The listing builds one solid part. Answer for the finished solid, in the listing's coordinates (mm). A direction names the side the tool comes from. Round coordinates to 2 decimals unless told otherwise and drop trailing zeros. Loops run counter-clockwise (first coordinate to the right, second up) from the corner with the lowest first, then second, coordinate; pieces in that order, holes last. Notation, with made-up numbers: (31, 52) -> (78, 52) arc R10 ccw to (78, 57) -> close; hole circle Ø7 at (-6, 67.5). An arc over 180 degrees is marked (long way). One line per question, with ' | ' between items.
from build123d import *

# Parameters (mm, degrees)
SKETCH_1_W          = 23
SKETCH_1_H          = 12
EXTRUDE_1_DEPTH     = 22
SKETCH_2_W          = 32
SKETCH_2_H          = 12
EXTRUDE_2_DEPTH     = 2.5
CUT_EXTRUDE_1_DEPTH = 25.103941586
EXTRUDE_3_DEPTH     = 5
SKETCH_5_R          = 2.5
EXTRUDE_4_DEPTH     = 4


with BuildPart() as part:
    # 草图1 → 凸台-拉伸1 (new body)
    with BuildSketch(Plane(origin=(0, 0, 0), x_dir=(1, 0, 0), z_dir=(0, 1, 0))):
        Rectangle(SKETCH_1_W, SKETCH_1_H)
    extrude(amount=EXTRUDE_1_DEPTH)

    # 草图2 → 凸台-拉伸2 (add)
    with BuildSketch(Plane(origin=(0, 17, 0), x_dir=(1, 0, 0), z_dir=(0, 1, 0))):
        Rectangle(SKETCH_2_W, SKETCH_2_H)
    extrude(amount=-EXTRUDE_2_DEPTH)

    # 草图3 → 切除-拉伸1 (cut, through all)
    with BuildSketch(Plane(origin=(0, 17, 0), x_dir=(1, 0, 0), z_dir=(0, 1, 0))):
        with BuildLine():
            Line((-16, 0.5), (-15.116025404, 0.5))
            ThreePointArc((-15.116025404, 0.5), (-13.25, 0), (-15.116025404, -0.5))
            Line((-15.116025404, -0.5), (-16, -0.5))
            Line((-16, -0.5), (-16, 0.5))
        make_face()
    cut_extrude_1 = extrude(amount=-CUT_EXTRUDE_1_DEPTH, mode=Mode.SUBTRACT)

    # 镜向1: 切除-拉伸1 across plane
    add(cut_extrude_1.mirror(Plane(origin=(0, 0, 0), x_dir=(0, 0, 1), z_dir=(1, 0, 0))), mode=Mode.SUBTRACT)

    # 草图4 → 凸台-拉伸3 (add)
    with BuildSketch(Plane(origin=(0, 22, 0), x_dir=(1, 0, 0), z_dir=(0, 1, 0))):
        with BuildLine():
            ThreePointArc((0.291208791, -2.978001703), (11.5, 0), (0.291208791, 2.978001703))
            ThreePointArc((0.291208791, 2.978001703), (0.017562524, 2.752601694), (-0.336734694, 2.765287296))
            ThreePointArc((-0.336734694, 2.765287296), (-4.5, 0), (-0.336734694, -2.765287296))
            ThreePointArc((-0.336734694, -2.765287296), (0.017562524, -2.752601694), (0.291208791, -2.978001703))
        make_face()
    extrude(amount=EXTRUDE_3_DEPTH)

    # 草图5 → 凸台-拉伸4 (add)
    with BuildSketch(Plane(origin=(0, 27, 0), x_dir=(1, 0, 0), z_dir=(0, 1, 0))):
        with Locations(Location((5.5, 0, 0), (0, 0, 90))):
            Circle(SKETCH_5_R)
    extrude(amount=EXTRUDE_4_DEPTH)


solid = part.part
Q1. Given pin 1 Ø3.5 at (y, z) = (6, 3) entering from -X; pin 2 Ø3.5 at (x, z) = (13.5, 2) entering from -Y; pin 3 Ø1.5 at (y, z) = (12.5, 2.5) entering from +X; pin 4 Ø1.2 at (x, z) = (14.25, 0) entering from -Y, each flat-ended and moving along its own axis, determine where each tip first touches the part or whether it passes through.
Numbers:
pin 1: x = -11.5 | pin 2: y = 14.5 | pin 3: x = 11.5 | pin 4: through
Q2. A cutting plane is placed at D-D on y = 7. Give the vertices of the cut face in (x, z).
Numbers:
outline: (-11.5, -6) -> (11.5, -6) -> (11.5, 6) -> (-11.5, 6) -> close
Q3. For faces 1 (the face through (-15.6, 15.8, 0.5)), 2 (the face through (11.5, 19, 0)), 3 (the face through (-11.5, 19, 0)), 4 (the face through (3, 27, -1)), determine the directions among +Z, -Z, +X, -X, +Y, -Y from which every point of the face is accessible in a straight line to the end or side of a thin tool.
Numbers:
face 1: -X, +Y, -Y | face 2: +Z, -Z, +X, +Y | face 3: +Z, -Z, -X, +Y | face 4: +Y
Q4. A cutting plane is placed at A-A on x = 14.25. Give the vertices of the cut face in (y, z).
Numbers:
outline: (14.5, -6) -> (17, -6) -> (17, -1) -> (14.5, -1) -> close; (14.5, 1) -> (17, 1) -> (17, 6) -> (14.5, 6) -> close
Q5. Find the intervals of material crossed by line 1 (X direction, y = 15.65, z = 0); line 2 (Y direction, x = -14.5, z = -3); line 3 (Y direction, x = -10.5, z = 1.5), in increasing order. Write a range as from..to.
Numbers:
line 1: -13.25..13.25 | line 2: 14.5..17 | line 3: 0..22
Q6. A cutting plane is placed at C-C on z = 3.5. Give the vertices of the cut face in (x, y).
Numbers:
outline: (-16, 14.5) -> (-11.5, 14.5) -> (-11.5, 0) -> (11.5, 0) -> (11.5, 14.5) -> (16, 14.5) -> (16, 17) -> (11.5, 17) -> (11.5, 22) -> (10.37, 22) -> (10.37, 27) -> (0.63, 27) -> (0.63, 22) -> (-11.5, 22) -> (-11.5, 17) -> (-16, 17) -> close
Q7. A cutting plane is placed at B-B on x = -1.5. Give the vertices of the cut face in (y, z).
Numbers:
outline: (0, -6) -> (22, -6) -> (22, -3) -> (27, -3) -> (27, 3) -> (22, 3) -> (22, 6) -> (0, 6) -> close
